from build123d import *

# Parameters (mm, degrees)
BOSS_EXTRUDE1_DEPTH = 24.13
SKETCH2_R           = 19.685
CUT_EXTRUDE1_DEPTH  = 49.26
SKETCH3_R           = 13.335
CUT_EXTRUDE2_DEPTH  = 64.5
SKETCH4_R           = 5.1435
CUT_EXTRUDE3_DEPTH  = 49.26


with BuildPart() as part:
    # Sketch1 → Boss-Extrude1 (new body, symmetric)
    with BuildSketch(Plane(origin=(0, 0, 0), x_dir=(1, 0, 0), z_dir=(0, 1, 0))):
        with BuildLine():
            Line((0, 31.75), (69.85, 31.75))
            ThreePointArc((69.85, 31.75), (79.502, 0), (69.85, -31.75))
            Line((69.85, -31.75), (0, -31.75))
            ThreePointArc((0, -31.75), (-31.75, 0), (0, 31.75))
        make_face()
    extrude(amount=BOSS_EXTRUDE1_DEPTH, both=True)

    # Sketch2 → Cut-Extrude1 (cut, through all)
    with BuildSketch(Plane(origin=(0, 24.13, 0), x_dir=(1, 0, 0), z_dir=(0, 1, 0))):
        Circle(SKETCH2_R)
    extrude(amount=-CUT_EXTRUDE1_DEPTH, mode=Mode.SUBTRACT)

    # Sketch3 → Cut-Extrude2 (cut, through all)
    with BuildSketch(Plane.XY.offset(31.75)):
        with Locations((43.18, 0)):
            Circle(SKETCH3_R)
    extrude(amount=-CUT_EXTRUDE2_DEPTH, mode=Mode.SUBTRACT)

    # Sketch4 → Cut-Extrude3 (cut, through all)
    with BuildSketch(Plane(origin=(0, 24.13, 0), x_dir=(1, 0, 0), z_dir=(0, 1, 0))):
        with Locations((69.85, 0)):
            Circle(SKETCH4_R)
    extrude(amount=-CUT_EXTRUDE3_DEPTH, mode=Mode.SUBTRACT)


solid = part.part
The model under review builds one solid part; all positions refer to its coordinate system, in mm. Coordinates: 2 decimals unless noted, no trailing zeros. Order: outer loops, then holes, each group sorted by start corner. A loop starts at its lowest first (then second) coordinate and runs counter-clockwise, first axis right, second up. Notation, with made-up numbers: (10.5, 32.5) -> (67.5, 32.5) arc R27 ccw to (67.5, 51.5) -> close; hole circle Ø7 at (89.5, -17). An arc over 180 degrees is marked (long way). Answer in a Markdown table with one row per item.
(1) Insertion check: pin 1 (6 mm diameter, centred on x = -10, y = -7.5, fed in from -Z); pin 2 (4 mm diameter, centred on y = -17, z = 1, fed in from -X). Each pin has a flat end and moves straight along its axis. Give the tip position at first contact, or say it passes through.
Answers:
| item | result |
|---|---|
| pin 1 | z = -30.97 |
| pin 2 | x = -31.75 |
(2) Consider section D-D (z = 11). Write out the cut boundary in (x, y) (3 decimals), plus the area to 3 significant figures.
Answers:
| item | result |
|---|---|
| outline | (-29.784, -24.13) -> (-16.325, -24.13) -> (-16.325, 24.13) -> (-29.784, 24.13) -> close; (16.325, -24.13) -> (78.431, -24.13) -> (78.431, 24.13) -> (16.325, 24.13) -> close; hole circle Ø26.67 at (43.18, 0) |
| area | 3,090 mm² |
(3) Wall thickness on line 1 along Z through (x, y) = (0, -12) (3 decimals); line 2 along X through (y, z) = (9.5, 15.5); line 3 along X through (y, z) = (-7, -12.5): over which ranges is each line inside the solid? List them lowest first.
Answers:
| item | result |
|---|---|
| line 1 | -31.75 to -19.685, 19.685 to 31.75 |
| line 2 | -27.71 to -12.13, 12.13 to 33.82, 52.54 to 77.36 |
| line 3 | -29.19 to -15.21, 15.21 to 31.83, 54.53 to 78.12 |
(4) Consider section A-A (z = 0). State how many separate pieces and enclosed holes the cut face has, plus the area to 3 significant figures.
Answers:
| item | result |
|---|---|
| separate pieces | 3 |
| enclosed holes | 1 |
| area | 2,410 mm² |
(5) Consider section B-B (x = 43.18). Write out the cut boundary in (y, z) (3 decimals), plus the area to 3 significant figures.
Answers:
| item | result |
|---|---|
| outline | (-24.13, -31.75) -> (-13.335, -31.75) -> (-13.335, 31.75) -> (-24.13, 31.75) -> close; (13.335, -31.75) -> (24.13, -31.75) -> (24.13, 31.75) -> (13.335, 31.75) -> close |
| area | 1,370 mm² |
(6) The part is to be moulded in two halves that separate along X. For faces 1 (the flat face through (37, 24.13, 0)), 2 (the cylindrical face through (64.71, 0.34, -0.23)), 3 (the cylindrical face through (79.5, 0.3, -0.5)), say which applies: +X half, -X half, draft (parallel to the pull), parting line (faces both ways), or undercut.
Answers:
| item | result |
|---|---|
| face 1 | draft |
| face 2 | undercut |
| face 3 | +X half |
